Read the model definition and answer for the solid it produces. Units are mm, in the model's axes. A direction names the side the tool comes from. Coordinates: 2 decimals unless noted, no trailing zeros. Write each loop counter-clockwise with the first axis right and the second up, starting at its lowest first coordinate (ties: lowest second). Pieces come first, ordered by that corner, then holes. Notation, with made-up numbers: (63.25, 66.25) -> (112.25, 66.25) arc R19 ccw to (112.25, 98.25) -> close; hole circle Ø10 at (-18.75, 78). An arc over 180 degrees is marked (long way). Answer in a Markdown table with one row per item. Add a question column.
Item 1: For a pull along Y with two mould halves and no side action, classify faces 1 (the face through (-1, -50, -20)), 2 (the face through (-1, 1, -30)), 3 (the face through (-50, -1, -20)) as +Y half, -Y half, draft (parallel to the pull), parting line (faces both ways), or undercut.
Item 2: Straight lines are drawn through the part: line 1 (Y direction, x = 12, z = -9.5); line 2 (X direction, y = -9.5, z = -11.5); line 3 (X direction, y = -12.5, z = -34). For each, find the intervals that lie inside material, in ascending order. Write a range as from..to.
Item 3: Section A-A on z = -12.5 is taken. Write down the section's boundary in (x, y), then the cut area to 3 significant figures.
Item 4: Section B-B on y = -30 is taken. Write down the section's boundary in (x, z).
Item 5: Section D-D on x = 21.5 is taken. Write down the section's boundary in (y, z), then the cut area to 3 significant figures.
Item 6: Given pin 1 Ø2 at (x, y) = (-4.5, -14) entering from +Z, flat-ended and moving along its own axis, determine where the tip first touches the part or whether it passes through.
Item 7: Which of the six approach directions +Z, -Z, +X, -X, +Y, -Y give full straight-line access (tool end or side, diameter ignored) to faces 4 (the face through (-1, 1, -40)), 5 (the face through (0, -11.058, -32))?
Item 8: Section C-C on x = 33.5 is taken. Write down the section's boundary in (y, z), then the cut area to 3 significant figures.
```python
from build123d import *

# Parameters (mm, degrees)
F0_W     = 100
F0_H     = 100
F1_DEPTH = 40
F2_W     = 88.950806
F2_H     = 88.116594
F3_DEPTH = 30
F4_W     = 50
F4_H     = 25
F5_DEPTH = 35


with BuildPart() as f1:
    # F0 (on Top) → F1 (new body)
    with BuildSketch(Plane.XY):
        Rectangle(F0_W, F0_H)
    extrude(amount=-F1_DEPTH)

    # F2 (on face) → F3 (cut)
    with BuildSketch(Plane.XY):
        Rectangle(F2_W, F2_H)
    extrude(amount=-F3_DEPTH, mode=Mode.SUBTRACT)

    # F4 (on Top) → F5 (cut)
    with BuildSketch(Plane.XY):
        with Locations((0, -23.558297)):
            Rectangle(F4_W, F4_H)
    extrude(amount=-F5_DEPTH, mode=Mode.SUBTRACT)


solid = f1.part
```
Results below:
| question | item | result |
|---|---|---|
| 1 | face 1 | -Y half |
| 1 | face 2 | undercut |
| 1 | face 3 | draft |
| 2 | line 1 | y = -50..-44.06, 44.06..50 |
| 2 | line 2 | x = -50..-44.48, 44.48..50 |
| 2 | line 3 | x = -50..-25, 25..50 |
| 3 | outline | (-50, -50) -> (50, -50) -> (50, 50) -> (-50, 50) -> close; hole (-44.48, -44.06) -> (44.48, -44.06) -> (44.48, 44.06) -> (-44.48, 44.06) -> close |
| 3 | area | 2,160 mm2 |
| 4 | outline | (-50, -40) -> (50, -40) -> (50, 0) -> (44.48, 0) -> (44.48, -30) -> (25, -30) -> (25, -35) -> (-25, -35) -> (-25, -30) -> (-44.48, -30) -> (-44.48, 0) -> (-50, 0) -> close |
| 5 | outline | (-50, -40) -> (50, -40) -> (50, 0) -> (44.06, 0) -> (44.06, -30) -> (-11.06, -30) -> (-11.06, -35) -> (-36.06, -35) -> (-36.06, -30) -> (-44.06, -30) -> (-44.06, 0) -> (-50, 0) -> close |
| 5 | area | 1,230 mm2 |
| 6 | pin 1 | stops at z = -35 |
| 7 | face 4 | -Z, +X, -X, +Y, -Y |
| 7 | face 5 | +Z |
| 8 | outline | (-50, -40) -> (50, -40) -> (50, 0) -> (44.06, 0) -> (44.06, -30) -> (-44.06, -30) -> (-44.06, 0) -> (-50, 0) -> close |
| 8 | area | 1,360 mm2 |
